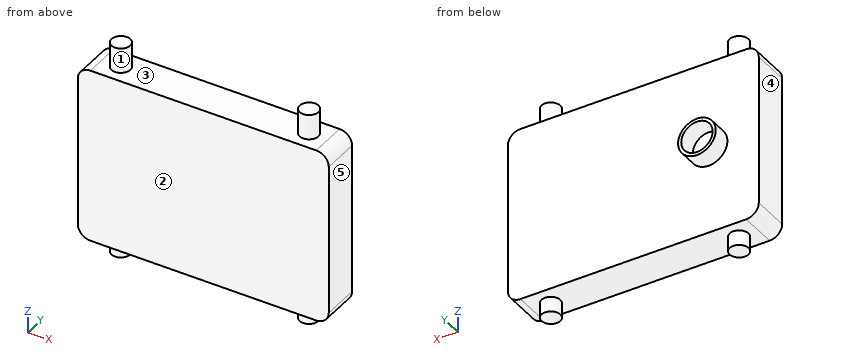
```python
from build123d import *

# Parameters (mm, degrees)
SKETCH1_W           = 200
SKETCH1_H           = 140
BOSS_EXTRUDE1_DEPTH = 30
FILLET1_R           = 10
SKETCH2_R           = 7.5
BOSS_EXTRUDE2_DEPTH = 20
BOSS_EXTRUDE3_START = 12
SKETCH4_R           = 7.5
BOSS_EXTRUDE3_DEPTH = 12
SKETCH6_R           = 15
SKETCH6_R_2         = 12.5
BOSS_EXTRUDE4_DEPTH = 45


with BuildPart() as part:
    # Sketch1 → Boss-Extrude1 (new body)
    with BuildSketch(Plane(origin=(0, 0, 0), x_dir=(1, 0, 0), z_dir=(0, 1, 0))):
        Rectangle(SKETCH1_W, SKETCH1_H)
    extrude(amount=BOSS_EXTRUDE1_DEPTH)

    # Fillet1
    fillet1_edges = [part.edges().sort_by_distance(p)[0] for p in [
        (100, 15, 70),
        (-100, 15, 70),
        (-100, 15, -70),
        (100, 15, -70),
    ]]
    fillet(fillet1_edges, radius=FILLET1_R)

    # Sketch2 → Boss-Extrude2 (add)
    with BuildSketch(Plane.XY.offset(70)):
        with Locations(Location((-75, 15, 0), (0, 0, 180))):
            Circle(SKETCH2_R)
        with Locations(Location((75, 15, 0), (0, 0, 180))):
            Circle(SKETCH2_R)
    extrude(amount=BOSS_EXTRUDE2_DEPTH)

    # Sketch4 → Boss-Extrude3 (add)
    with BuildSketch(Plane(origin=(0, 0, -70), x_dir=(-1, 0, 0), z_dir=(0, 0, -1)).offset(BOSS_EXTRUDE3_START)):
        with Locations((-75, 15)):
            Circle(SKETCH4_R)
        with Locations((75, 15)):
            Circle(SKETCH4_R)
    extrude(amount=-BOSS_EXTRUDE3_DEPTH)

    # Sketch6 → Boss-Extrude4 (add)
    with BuildSketch(Plane.XZ):
        with Locations(Location((-60, 0, 0), (0, 0, 270))):
            Circle(SKETCH6_R)
        with Locations(Location((-60, 0, 0), (0, 0, 270))):
            Circle(SKETCH6_R_2, mode=Mode.SUBTRACT)
    extrude(amount=-BOSS_EXTRUDE4_DEPTH)


solid = part.part
```
Work out the finished part from the listing and answer in its coordinate system (mm). Face numbers are marked on the shaded views. A direction names the side the tool comes from. Give positions to 0.01 mm unless a question says otherwise; leave off trailing zeros. Order: outer loops, then holes, each group sorted by start corner. A loop starts at its lowest first (then second) coordinate and runs counter-clockwise, first axis right, second up. Notation, with made-up numbers: (85, 85) -> (91, 85) arc R32 ccw to (91, 124) -> close; hole circle Ø8 at (-26.5, -21). An arc over 180 degrees is marked (long way). Answer as CSV lines item,"result". Start each with the question number.
(1) Consider line 1 along X through (y, z) = (33, 0); line 2 along Y through (x, z) = (-10, 33); line 3 along Z through (x, y) = (37.5, 24). Determine where each line is inside the solid, lowest interval first.
(2) Each of these flat-tipped pins is pushed along its axis until it touches: pin 1 Ø15 at (x, z) = (-60, 0) entering from +Y; pin 2 Ø8 at (x, y) = (41.5, 10) entering from -Z; pin 3 Ø6 at (x, y) = (-72, 40) entering from +Z; pin 4 Ø1.5 at (x, y) = (-72.5, 7.5) entering from +Z. Where does it stop, or does it pass through?
(3) Section B-B, the plane x = -60 is taken. Write down the section's boundary in (y, z).
(4) Section A-A, the plane z = 0 is taken. Write down the section's boundary in (x, y), plus the area to 4 significant figures.
(5) Which of the six approach directions +Z, -Z, +X, -X, +Y, -Y give full straight-line access (tool end or side, diameter ignored) to the marked faces 1 and 2?
(6) For a pull along X with two mould halves and no side action, classify the marked faces 3, 4 and 5 as released by +X, released by -X, zero draft, split by the parting line, or undercut.
(7) Section D-D, the plane y = 15 is taken. Write down the section's boundary in (x, z), plus the area to 3 significant figures.
(8) Section C-C, the plane y = 25 is taken. Write down the section's boundary in (x, z).
Entries:
1,line 1,"-75 to -72.5, -47.5 to -45"
1,line 2,"0 to 30"
1,line 3,"-70 to 70"
2,pin 1,"y = 30"
2,pin 2,"z = -70"
2,pin 3,"z = 12"
2,pin 4,"z = 90"
3,outline,"(0, -70) -> (30, -70) -> (30, -15) -> (45, -15) -> (45, -12.5) -> (30, -12.5) -> (30, 12.5) -> (45, 12.5) -> (45, 15) -> (30, 15) -> (30, 70) -> (0, 70) -> close"
4,outline,"(-100, 0) -> (100, 0) -> (100, 30) -> (-45, 30) -> (-45, 45) -> (-47.5, 45) -> (-47.5, 30) -> (-72.5, 30) -> (-72.5, 45) -> (-75, 45) -> (-75, 30) -> (-100, 30) -> close"
4,area,"6,075 mm²"
5,face 1,"+Z"
5,face 2,"+Z, -Z, +X, -X, -Y"
6,face 3,"undercut"
6,face 4,"released by -X"
6,face 5,"released by +X"
7,outline,"(-100, -60) arc R10 ccw to (-90, -70) -> (-82.5, -70) -> (-82.5, -82) -> (-67.5, -82) -> (-67.5, -70) -> (67.5, -70) -> (67.5, -82) -> (82.5, -82) -> (82.5, -70) -> (90, -70) arc R10 ccw to (100, -60) -> (100, 60) arc R10 ccw to (90, 70) -> (82.5, 70) -> (82.5, 90) -> (67.5, 90) -> (67.5, 70) -> (-67.5, 70) -> (-67.5, 90) -> (-82.5, 90) -> (-82.5, 70) -> (-90, 70) arc R10 ccw to (-100, 60) -> close"
7,area,"28,900 mm²"
8,outline,"(-100, -60) arc R10 ccw to (-90, -70) -> (90, -70) arc R10 ccw to (100, -60) -> (100, 60) arc R10 ccw to (90, 70) -> (-90, 70) arc R10 ccw to (-100, 60) -> close"
